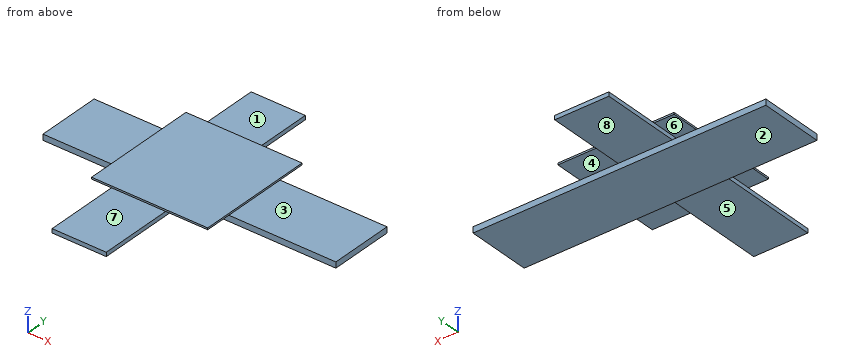
from build123d import *

# Parameters (mm, degrees)
F0_W     = 127.1624974906
F0_H     = 27.8577823192
F1_DEPTH = 2.54
F2_W     = 23.5141962767
F2_H     = 27.8577823192
F2_H_2   = 46.019657515
F2_H_3   = 34.5669230446
F3_DEPTH = 1.778
F4_W     = 18.2572918436
F4_H     = 51.4373374962
F4_W_2   = 23.5141962767
F4_W_3   = 8.6478181183
F5_DEPTH = 0.762


with BuildPart() as f1:
    # F0 (on Top) → F1 (new body)
    with BuildSketch(Plane.XY):
        with Locations((-14.2351035029, 13.9288911596)):
            Rectangle(F0_W, F0_H)
    extrude(amount=F1_DEPTH)

    # F2 (on face) → F3 (join)
    with BuildSketch(Plane.XY.offset(2.54)):
        with Locations((-25.4345647991, 13.9288911596)):
            Rectangle(F2_W, F2_H)
        with Locations((-25.4345647991, -23.0098287575)):
            Rectangle(F2_W, F2_H_2)
        with Locations((-25.4345647991, 45.1412438415)):
            Rectangle(F2_W, F2_H_3)
    extrude(amount=F3_DEPTH)

    # F4 (on face) → F5 (join)
    with BuildSketch(Plane.XY.offset(4.318)):
        with Locations((-4.5488207389, 12.0593749848)):
            Rectangle(F4_W, F4_H)
        with Locations((-25.4345647991, 12.0593749848)):
            Rectangle(F4_W_2, F4_H)
        with Locations((-41.5155719966, 12.0593749848)):
            Rectangle(F4_W_3, F4_H)
    extrude(amount=F5_DEPTH)


solid = f1.part
Check sheet for the modelled part. Datum: model origin and axes. Units: mm. Face numbers are marked on the shaded views. A direction names the side the tool comes from. Coordinates: 2 decimals unless noted, no trailing zeros. Loops run counter-clockwise (first coordinate to the right, second up) from the corner with the lowest first, then second, coordinate; pieces in that order, holes last. Notation, with made-up numbers: (6, -25) -> (56, -25) arc R17 cw to (56, -10) -> close; hole circle Ø8 at (84.5, 77). An arc over 180 degrees is marked (long way). Answer in a Markdown table with one row per item.
1. Sectioned sample at D-D, the plane y = 13.5. Record the boundary of the cut face in (x, z).
Check values:
| item | result |
|---|---|
| outline | (-77.82, 0) -> (49.35, 0) -> (49.35, 2.54) -> (-13.68, 2.54) -> (-13.68, 4.32) -> (4.58, 4.32) -> (4.58, 5.08) -> (-45.84, 5.08) -> (-45.84, 4.32) -> (-37.19, 4.32) -> (-37.19, 2.54) -> (-77.82, 2.54) -> close |
2. Access from +Z, -Z, +X, -X, +Y, -Y to the whole of each face (thin tool, end or side, straight path). Record for the marked faces 4, 5, 6, 7 and 8.
Check values:
| item | result |
|---|---|
| face 4 | +X, +Y, -Y |
| face 5 | -Z, +X, -X, -Y |
| face 6 | -X, +Y, -Y |
| face 7 | +Z, +X, -X, -Y |
| face 8 | -Z, +X, -X, +Y |
3. Sectioned sample at C-C, the plane z = 1.6. Record the boundary of the cut face in (x, y).
Check values:
| item | result |
|---|---|
| outline | (-77.82, 0) -> (49.35, 0) -> (49.35, 27.86) -> (-77.82, 27.86) -> close |
4. Release check for a two-part mould opening along Z. For the marked faces 1, 2 and 3 record: released by +Z, released by -Z, zero draft, split by the parting line, or undercut.
Check values:
| item | result |
|---|---|
| face 1 | released by +Z |
| face 2 | released by -Z |
| face 3 | undercut |
5. Sectioned sample at B-B, the plane y = 34. Record the boundary of the cut face in (x, z).
Check values:
| item | result |
|---|---|
| outline | (-45.84, 4.32) -> (-37.19, 4.32) -> (-37.19, 2.54) -> (-13.68, 2.54) -> (-13.68, 4.32) -> (4.58, 4.32) -> (4.58, 5.08) -> (-45.84, 5.08) -> close |
6. Material ranges on line 1 along Y through (x, z) = (-21, 0.85); line 2 along X through (y, z) = (7.5, 3.85); line 3 along X through (y, z) = (12.5, 4.5), recorded low to high. Write a range as [from, to].
Check values:
| item | result |
|---|---|
| line 1 | y = [0, 27.86] |
| line 2 | x = [-37.19, -13.68] |
| line 3 | x = [-45.84, 4.58] |
7. Sectioned sample at A-A, the plane x = 1. Record the boundary of the cut face in (y, z), then the cut area to 3 significant figures.
Check values:
| item | result |
|---|---|
| outline | (-13.66, 4.32) -> (37.78, 4.32) -> (37.78, 5.08) -> (-13.66, 5.08) -> close; (0, 0) -> (27.86, 0) -> (27.86, 2.54) -> (0, 2.54) -> close |
| area | 110 mm2 |
8. Go/stop test with flat-tipped pins: pin 1 (0.6 mm diameter, centred on x = -14, z = 5, fed in from +Y); pin 2 (1 mm diameter, centred on y = -10.5, z = 2, fed in from +X); pin 3 (2 mm diameter, centred on x = -22.5, z = 1.5, fed in from +Y); pin 4 (0.8 mm diameter, centred on y = 22.5, z = 5, fed in from +X). Record where each tip stops, or that it passes through.
Check values:
| item | result |
|---|---|
| pin 1 | stops at y = 37.78 |
| pin 2 | passes through |
| pin 3 | stops at y = 27.86 |
| pin 4 | stops at x = 4.58 |
